Design review of the part built by this model. Coordinates are the model's own, in mm. Face numbers are marked on the shaded views. A direction names the side the tool comes from. Coordinates: 2 decimals unless noted, no trailing zeros. Order: outer loops, then holes, each group sorted by start corner. A loop starts at its lowest first (then second) coordinate and runs counter-clockwise, first axis right, second up. Notation, with made-up numbers: M 81.25,37 L 130.25,37 A16 cw 130.25,56 Z; hole C -13,38.5 d5. An arc over 180 degrees is marked long. Use CSV: the item, a comma, the result in double quotes.
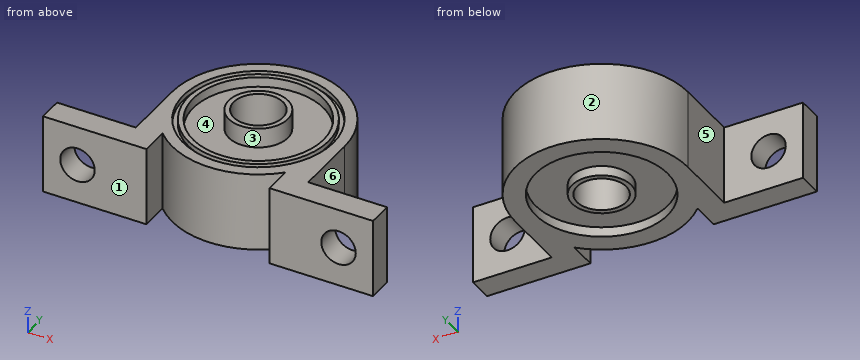
```python
from build123d import *

# Parameters (mm, degrees)
SKETCH_1_R          = 5
EXTRUDE_1_DEPTH     = 16
SKETCH_2_R          = 6
SKETCH_2_R_2        = 5
EXTRUDE_2_DEPTH     = 2
CUT_EXTRUDE_START   = -2
SKETCH_3_R          = 13.227089176
SKETCH_3_R_2        = 6
CUT_EXTRUDE_1_DEPTH = 2
SKETCH_4_R          = 13.402399482
SKETCH_4_R_2        = 6
CUT_EXTRUDE_2_DEPTH = 2
SKETCH_5_R          = 15.227089176
SKETCH_5_R_2        = 14.227089176
CUT_EXTRUDE_3_DEPTH = 1
SKETCH_6_R          = 3.5
CUT_EXTRUDE_4_DEPTH = 10


with BuildPart() as part:
    # 草图1 → 凸台-拉伸1 (new body)
    with BuildSketch(Plane.XY):
        with BuildLine():
            Line((-12.5, -18), (-33.5, -18))
            Line((-33.5, -18), (-33.5, -13))
            Line((-33.5, -13), (-17.5, -13))
            Line((-17.5, -13), (-17.5, 0))
            ThreePointArc((-17.5, 0), (0, 17.5), (17.5, 0))
            Line((17.5, 0), (17.5, -13))
            Line((17.5, -13), (33.5, -13))
            Line((33.5, -13), (33.5, -18))
            Line((33.5, -18), (12.5, -18))
            Line((12.5, -18), (12.5, -12.247448714))
            ThreePointArc((12.5, -12.247448714), (0, -17.5), (-12.5, -12.247448714))
            Line((-12.5, -12.247448714), (-12.5, -18))
        make_face()
        Circle(SKETCH_1_R, mode=Mode.SUBTRACT)
    extrude(amount=EXTRUDE_1_DEPTH)

    # 草图2 → 凸台-拉伸2 (add)
    with BuildSketch(Plane.XY.offset(16)):
        Circle(SKETCH_2_R)
        Circle(SKETCH_2_R_2, mode=Mode.SUBTRACT)
    extrude(amount=EXTRUDE_2_DEPTH)

    # 草图3 → 切除-拉伸1 (cut)
    with BuildSketch(Plane.XY.offset(16).offset(CUT_EXTRUDE_START)):
        Circle(SKETCH_3_R)
        Circle(SKETCH_3_R_2, mode=Mode.SUBTRACT)
    extrude(amount=CUT_EXTRUDE_1_DEPTH, mode=Mode.SUBTRACT)

    # 草图4 → 切除-拉伸2 (cut)
    with BuildSketch(Plane(origin=(0, 0, 0), x_dir=(-1, 0, 0), z_dir=(0, 0, -1))):
        Circle(SKETCH_4_R)
        with Locations(Location((0, 0, 0), (0, 0, 180))):
            Circle(SKETCH_4_R_2, mode=Mode.SUBTRACT)
    extrude(amount=-CUT_EXTRUDE_2_DEPTH, mode=Mode.SUBTRACT)

    # 草图5 → 切除-拉伸3 (cut)
    with BuildSketch(Plane.XY.offset(16)):
        Circle(SKETCH_5_R)
        Circle(SKETCH_5_R_2, mode=Mode.SUBTRACT)
    extrude(amount=-CUT_EXTRUDE_3_DEPTH, mode=Mode.SUBTRACT)

    # 草图6 → 切除-拉伸4 (cut)
    with BuildSketch(Plane.XZ.offset(18)):
        with Locations((26.5, 8)):
            Circle(SKETCH_6_R)
        with Locations(Location((-26.5, 8, 0), (0, 0, 270))):
            Circle(SKETCH_6_R)
    extrude(amount=-CUT_EXTRUDE_4_DEPTH, mode=Mode.SUBTRACT)


solid = part.part
```
(1) The part is to be moulded in two halves that separate along X. For the marked faces 1, 2 and 3, say which applies: pulls with the +X half, pulls with the -X half, needs draft (parallel to the pull), parting line crosses it, or undercut.
The answers:
face 1,"needs draft"
face 2,"parting line crosses it"
face 3,"undercut"
(2) Add section C-C on z = 12.5. State the section outline as (x, y) points.
The answers:
outline,"M -33.5,-18 L -12.5,-18 L -12.5,-12.25 A17.5 ccw 12.5,-12.25 L 12.5,-18 L 33.5,-18 L 33.5,-13 L 17.5,-13 L 17.5,0 A17.5 ccw -17.5,0 L -17.5,-13 L -33.5,-13 Z; hole C 0,0 d10"
(3) Add section B-B on x = -26.5. State the section outline as (y, z) points.
The answers:
outline,"M -18,0 L -13,0 L -13,4.5 L -18,4.5 Z; M -18,11.5 L -13,11.5 L -13,16 L -18,16 Z"
(4) Wall thickness on probe 1 along Y at (x, z) = (0, 15.6); probe 2 along Y at (x, z) = (0, 1.55); probe 3 along X at (y, z) = (-16, 2.75): over which ranges is each line inside the solid? List them lowest first.
The answers:
probe 1,"y = -17.5 to -15.23, -14.23 to -13.23, -6 to -5, 5 to 6, 13.23 to 14.23, 15.23 to 17.5"
probe 2,"y = -17.5 to -13.4, -6 to -5, 5 to 6, 13.4 to 17.5"
probe 3,"x = -33.5 to -12.5, -7.09 to 7.09, 12.5 to 33.5"
(5) Add section A-A on z = 8. State the section outline as (x, y) points.
The answers:
outline,"M -33.5,-18 L -30,-18 L -30,-13 L -33.5,-13 Z; M -23,-18 L -12.5,-18 L -12.5,-12.25 A17.5 ccw 12.5,-12.25 L 12.5,-18 L 23,-18 L 23,-13 L 17.5,-13 L 17.5,0 A17.5 ccw -17.5,0 L -17.5,-13 L -23,-13 Z; M 30,-18 L 33.5,-18 L 33.5,-13 L 30,-13 Z; hole C 0,0 d10"
(6) For the marked faces 4, 5 and 6, list the 3-axis set-ups (+Z, -Z, +X, -X, +Y, -Y) from which the entire face can be reached by the end or side of a thin tool; tool diameter is ignored.
The answers:
face 4,"+Z"
face 5,"+Z, -Z, -X, +Y"
face 6,"+Z, -Z, +X, +Y"
(7) Add section D-D on y = -7. State the section outline as (x, z) points.
The answers:
outline,"M -17.5,0 L -11.43,0 L -11.43,2 L 11.43,2 L 11.43,0 L 17.5,0 L 17.5,16 L 13.52,16 L 13.52,15 L 12.39,15 L 12.39,16 L 11.22,16 L 11.22,14 L -11.22,14 L -11.22,16 L -12.39,16 L -12.39,15 L -13.52,15 L -13.52,16 L -17.5,16 Z"
(8) Clearance check with flat-ended pins moving along their axes: P1, Ø9, axis at x = -26.5, z = 8, coming from the +Y side; P2, Ø10.5, axis at y = -5.5, z = 7, coming from the -X side; P3, Ø4, axis at x = 23.5, y = -13.5, coming from the +Z side. State where each tip first meets the part, or that it passes through.
The answers:
P1,"stops at y = -13"
P2,"stops at x = -17.5"
P3,"stops at z = 16"
